The model under review builds one solid part; all positions refer to its coordinate system, in mm. Round coordinates to 2 decimals unless told otherwise and drop trailing zeros. Loops run counter-clockwise (first coordinate to the right, second up) from the corner with the lowest first, then second, coordinate; pieces in that order, holes last. Notation, with made-up numbers: (-39, -35.5) -> (-15, -35.5) arc R20 ccw to (-15, -12.5) -> close; hole circle Ø9 at (27.5, 72). An arc over 180 degrees is marked (long way). Return JSON: item names as keys, results as strings. Group by question number.
Autodesk Inventor part; units mm, degrees
ref_plane "YZ Plane" through (0, 0, 0) normal (1, 0, 0) x (0, 1, 0)
ref_plane "XZ Plane" through (0, 0, 0) normal (0, 1, 0) x (-1, 0, 0)
ref_plane "XY Plane" through (0, 0, 0) normal (0, 0, 1) x (1, 0, 0)
sketch "Sketch1" plane through (0, 0, 0) normal (0, 1, 0) x (-1, 0, 0)
  line L0 (10, 0) -> (15, 0)
  line L1 (25, -10) -> (25, -40)
  line L2 (15, -50) -> (10, -50)
  line L3 (0, -40) -> (0, -10)
  arc A0 (25, -2) -> (23, 0) centre (23, -2) ccw
  arc A1 (25, -10) -> (15, 0) centre (15, -10) ccw
  arc A2 (10, 0) -> (0, -10) centre (10, -10) ccw
  arc A3 (0, -40) -> (10, -50) centre (10, -40) ccw
  arc A4 (15, -50) -> (25, -40) centre (15, -40) ccw
  point P0 (0, 0)
  point P1 (25, -50)
  point P2 (25, 0)
  point P3 (0, -50)
  dimension "d0" = 25
  dimension "d1" = 50
  dimension "d2" = 2
  dimension "d3" = 10
extrude "Extrusion1" add sketch "Sketch1" along normal blind 1
properties part number "popsicle stick"
1. We need section B-B, the plane x = -3.5. Write out the cut boundary in (y, z).
2. Wall thickness on line 1 (X direction, y = 0.15, z = -42); line 2 (Z direction, x = -2, y = 0.9); line 3 (X direction, y = 0.7, z = -3): over which ranges is each line inside the solid? List them lowest first.
3. We need section C-C, the plane z = -44. Write out the cut boundary in (x, y), then the cut area to 3 significant figures.
4. We need section A-A, the plane y = 0.35. Write out the cut boundary in (x, z).
5. Draft analysis for pull direction Y (two halves, no side actions). For faces 1 (the face through (-2.85, 0.49, -3.01)), 2 (the face through (-12, 0, -25)), 3 (the face through (-12, 1, -25)), state which applies: pulls with the +Y half, pulls with the -Y half, needs draft (parallel to the pull), parting line crosses it, or undercut.
Check sheet entries:
{
 "1": {"outline": "(0, -47.6) -> (1, -47.6) -> (1, -2.4) -> (0, -2.4) -> close"},
 "2": {"line 1": "x = -24.8 to -0.2", "line 2": "z = -46 to -4", "line 3": "x = -22.14 to -2.86"},
 "3": {"outline": "(-24.17, 0) -> (-0.83, 0) -> (-0.83, 1) -> (-24.17, 1) -> close", "area": "23.3 mm²"},
 "4": {"outline": "(-25, -40) arc R10 ccw to (-15, -50) -> (-10, -50) arc R10 ccw to (0, -40) -> (0, -10) arc R10 ccw to (-10, 0) -> (-15, 0) arc R10 ccw to (-25, -10) -> close"},
 "5": {"face 1": "needs draft", "face 2": "pulls with the -Y half", "face 3": "pulls with the +Y half"}
}
